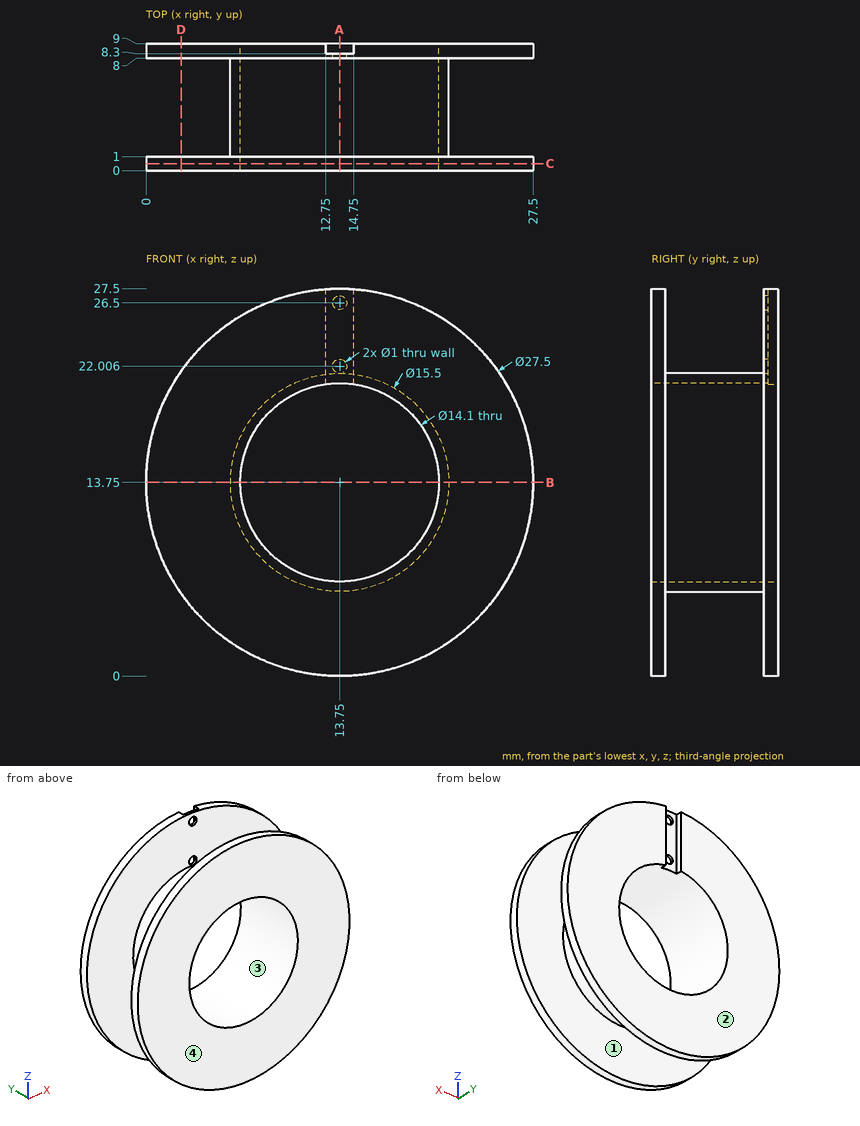
Study the drawing (mm; zero at the part's minimum x, y, z) and answer. A direction names the side the tool comes from. Round coordinates to 2 decimals unless told otherwise and drop trailing zeros. Loops run counter-clockwise (first coordinate to the right, second up) from the corner with the lowest first, then second, coordinate; pieces in that order, holes last. Notation, with made-up numbers: (66, 22.5) - (117, 22.5) arc R7 cw to (117, 26.5) - close; hole circle Ø11 at (25.5, 26.25). An arc over 180 degrees is marked (long way). Use one line per item in the form item = value. Start each with the question number.
1. The part is cut by section B-B on z = 13.75. Determine the outline of the cut face in (x, y).
2. The part is cut by section C-C on y = 0.5. Determine the outline of the cut face in (x, z).
3. The part is cut by section A-A on x = 13.75. Give the number of separate pieces and of enclosed holes in the cut face.
4. Given pin 1 Ø2 at (y, z) = (5, 7) entering from +X (1 decimal); pin 2 Ø3 at (y, z) = (5, 18) entering from -X; pin 3 Ø1.5 at (y, z) = (7.5, 17) entering from -X, each flat-ended and moving along its own axis, determine where each tip first touches the part or whether it passes through.
5. Consider line 1 (Y direction, x = 25.5, z = 13); line 2 (Z direction, x = 18.5, y = 6) (1 decimal); line 3 (X direction, y = 2, z = 13.75). Determine where each line is inside the solid, lowest interval first. Write a range as [from, to].
6. The part is cut by section D-D on x = 2.5. Determine the outline of the cut face in (y, z).
7. For a pull along Z with two mould halves and no side action, classify the marked faces 3 and 4 as pulls with the +Z half, pulls with the -Z half, needs draft (parallel to the pull), parting line crosses it, or undercut.
8. A tool of negligible diameter and unlimited length cuts with its end or side. For the marked faces 1 and 2, from which of +Z, -Z, +X, -X, +Y, -Y can it reach the whole face along a straight path? Write none if from no direction.
Geometry check:
q1.outline = (0, 0) - (6.7, 0) - (6.7, 9) - (0, 9) - (0, 8) - (6, 8) - (6, 1) - (0, 1) - close; (20.8, 0) - (27.5, 0) - (27.5, 1) - (21.5, 1) - (21.5, 8) - (27.5, 8) - (27.5, 9) - (20.8, 9) - close
q2.outline = circle Ø27.5 at (13.75, 13.75); hole circle Ø14.1 at (13.75, 13.75)
q3.separate_pieces = 4
q3.enclosed_holes = 0
q4.pin_1 = 18.9
q4.pin_2 = 6.5
q4.pin_3 = 0.27
q5.line_1 = [0, 1], [8, 9]
q5.line_2 = [7.6, 8.5], [19, 19.9]
q5.line_3 = [6, 6.7], [20.8, 21.5]
q6.outline = (0, 5.84) - (1, 5.84) - (1, 21.66) - (0, 21.66) - close; (8, 5.84) - (9, 5.84) - (9, 21.66) - (8, 21.66) - close
q7.face_3 = undercut
q7.face_4 = needs draft
q8.face_1 = none
q8.face_2 = +Z, -Z, +X, -X, +Y
